from build123d import *

# Parameters (mm, degrees)
ESQUISSE1_W        = 265
ESQUISSE1_H        = 227
ESQUISSE1_R        = 6.5
ESQUISSE1_R_2      = 1.75
ESQUISSE1_R_3      = 1.749999999
ESQUISSE1_W_2      = 191
ESQUISSE1_H_2      = 156.859849262
ESQUISSE1_W_3      = 17
ESQUISSE1_H_3      = 80
BOSS_EXTRU_1_DEPTH = 6


with BuildPart() as part:
    # Esquisse1 → Boss.-Extru.1 (new body)
    with BuildSketch(Plane(origin=(0, 0, 0), x_dir=(1, 0, 0), z_dir=(0, 1, 0))):
        with Locations((132.5, -113.5)):
            Rectangle(ESQUISSE1_W, ESQUISSE1_H)
        with Locations(Location((246.5, -113.5, 0), (0, 0, 270))):
            Circle(ESQUISSE1_R, mode=Mode.SUBTRACT)
        with Locations(Location((246.5, -103.5, 0), (0, 0, 270))):
            Circle(ESQUISSE1_R_2, mode=Mode.SUBTRACT)
        with Locations(Location((253.571068024, -106.4289324, 0), (0, 0, 270))):
            Circle(ESQUISSE1_R_2, mode=Mode.SUBTRACT)
        with Locations(Location((256.5, -113.5, 0), (0, 0, 270))):
            Circle(ESQUISSE1_R_2, mode=Mode.SUBTRACT)
        with Locations(Location((253.571067812, -120.571067812, 0), (0, 0, 270))):
            Circle(ESQUISSE1_R_2, mode=Mode.SUBTRACT)
        with Locations(Location((246.5, -123.5, 0), (0, 0, 270))):
            Circle(ESQUISSE1_R_2, mode=Mode.SUBTRACT)
        with Locations(Location((239.428932188, -120.571067812, 0), (0, 0, 270))):
            Circle(ESQUISSE1_R_2, mode=Mode.SUBTRACT)
        with Locations(Location((236.5, -113.5, 0), (0, 0, 270))):
            Circle(ESQUISSE1_R_2, mode=Mode.SUBTRACT)
        with Locations(Location((239.42893238, -106.428931957, 0), (0, 0, 270))):
            Circle(ESQUISSE1_R_3, mode=Mode.SUBTRACT)
        with Locations(Location((259.935029054, -100.064971369, 0), (0, 0, 270))):
            Circle(ESQUISSE1_R_2, mode=Mode.SUBTRACT)
        with Locations(Location((259.935028843, -126.935028843, 0), (0, 0, 270))):
            Circle(ESQUISSE1_R_2, mode=Mode.SUBTRACT)
        with Locations(Location((233.064971369, -100.064970946, 0), (0, 0, 270))):
            Circle(ESQUISSE1_R_2, mode=Mode.SUBTRACT)
        with Locations(Location((233.064971157, -126.935028843, 0), (0, 0, 270))):
            Circle(ESQUISSE1_R_2, mode=Mode.SUBTRACT)
        with Locations(Location((132.5, -209.464962315, 0), (0, 0, 270))):
            Circle(ESQUISSE1_R, mode=Mode.SUBTRACT)
        with Locations(Location((132.5, -199.464962315, 0), (0, 0, 270))):
            Circle(ESQUISSE1_R_2, mode=Mode.SUBTRACT)
        with Locations(Location((139.571068024, -202.393894715, 0), (0, 0, 270))):
            Circle(ESQUISSE1_R_2, mode=Mode.SUBTRACT)
        with Locations(Location((142.5, -209.464962315, 0), (0, 0, 270))):
            Circle(ESQUISSE1_R_2, mode=Mode.SUBTRACT)
        with Locations(Location((139.571067812, -216.536030127, 0), (0, 0, 270))):
            Circle(ESQUISSE1_R_2, mode=Mode.SUBTRACT)
        with Locations(Location((132.5, -219.464962315, 0), (0, 0, 270))):
            Circle(ESQUISSE1_R_2, mode=Mode.SUBTRACT)
        with Locations(Location((125.428932188, -216.536030127, 0), (0, 0, 270))):
            Circle(ESQUISSE1_R_2, mode=Mode.SUBTRACT)
        with Locations(Location((122.5, -209.464962315, 0), (0, 0, 270))):
            Circle(ESQUISSE1_R_2, mode=Mode.SUBTRACT)
        with Locations(Location((125.42893238, -202.393894272, 0), (0, 0, 270))):
            Circle(ESQUISSE1_R_3, mode=Mode.SUBTRACT)
        with Locations(Location((145.935029054, -196.029933685, 0), (0, 0, 270))):
            Circle(ESQUISSE1_R_2, mode=Mode.SUBTRACT)
        with Locations(Location((145.935028843, -222.899991158, 0), (0, 0, 270))):
            Circle(ESQUISSE1_R_2, mode=Mode.SUBTRACT)
        with Locations(Location((119.064971369, -196.029933261, 0), (0, 0, 270))):
            Circle(ESQUISSE1_R_2, mode=Mode.SUBTRACT)
        with Locations(Location((119.064971157, -222.899991158, 0), (0, 0, 270))):
            Circle(ESQUISSE1_R_2, mode=Mode.SUBTRACT)
        with Locations(Location((18.513965978, -113.5, 0), (0, 0, 270))):
            Circle(ESQUISSE1_R, mode=Mode.SUBTRACT)
        with Locations(Location((18.513965978, -103.5, 0), (0, 0, 270))):
            Circle(ESQUISSE1_R_2, mode=Mode.SUBTRACT)
        with Locations(Location((25.585034002, -106.4289324, 0), (0, 0, 270))):
            Circle(ESQUISSE1_R_2, mode=Mode.SUBTRACT)
        with Locations(Location((28.513965978, -113.5, 0), (0, 0, 270))):
            Circle(ESQUISSE1_R_2, mode=Mode.SUBTRACT)
        with Locations(Location((25.58503379, -120.571067812, 0), (0, 0, 270))):
            Circle(ESQUISSE1_R_2, mode=Mode.SUBTRACT)
        with Locations(Location((18.513965978, -123.5, 0), (0, 0, 270))):
            Circle(ESQUISSE1_R_2, mode=Mode.SUBTRACT)
        with Locations(Location((11.442898166, -120.571067812, 0), (0, 0, 270))):
            Circle(ESQUISSE1_R_2, mode=Mode.SUBTRACT)
        with Locations(Location((8.513965978, -113.5, 0), (0, 0, 270))):
            Circle(ESQUISSE1_R_2, mode=Mode.SUBTRACT)
        with Locations(Location((11.442898358, -106.428931957, 0), (0, 0, 270))):
            Circle(ESQUISSE1_R_3, mode=Mode.SUBTRACT)
        with Locations(Location((31.948995033, -100.064971369, 0), (0, 0, 270))):
            Circle(ESQUISSE1_R_2, mode=Mode.SUBTRACT)
        with Locations(Location((31.948994821, -126.935028843, 0), (0, 0, 270))):
            Circle(ESQUISSE1_R_2, mode=Mode.SUBTRACT)
        with Locations(Location((5.078937347, -100.064970946, 0), (0, 0, 270))):
            Circle(ESQUISSE1_R_2, mode=Mode.SUBTRACT)
        with Locations(Location((5.078937136, -126.935028843, 0), (0, 0, 270))):
            Circle(ESQUISSE1_R_2, mode=Mode.SUBTRACT)
        with Locations(Location((132.5, -18.5, 0), (0, 0, 270))):
            Circle(ESQUISSE1_R, mode=Mode.SUBTRACT)
        with Locations(Location((132.5, -8.5, 0), (0, 0, 270))):
            Circle(ESQUISSE1_R_2, mode=Mode.SUBTRACT)
        with Locations(Location((139.571068024, -11.4289324, 0), (0, 0, 270))):
            Circle(ESQUISSE1_R_2, mode=Mode.SUBTRACT)
        with Locations(Location((142.5, -18.5, 0), (0, 0, 270))):
            Circle(ESQUISSE1_R_2, mode=Mode.SUBTRACT)
        with Locations(Location((139.571067812, -25.571067812, 0), (0, 0, 270))):
            Circle(ESQUISSE1_R_2, mode=Mode.SUBTRACT)
        with Locations(Location((132.5, -28.5, 0), (0, 0, 270))):
            Circle(ESQUISSE1_R_2, mode=Mode.SUBTRACT)
        with Locations(Location((125.428932188, -25.571067812, 0), (0, 0, 270))):
            Circle(ESQUISSE1_R_2, mode=Mode.SUBTRACT)
        with Locations(Location((122.5, -18.5, 0), (0, 0, 270))):
            Circle(ESQUISSE1_R_2, mode=Mode.SUBTRACT)
        with Locations(Location((125.42893238, -11.428931957, 0), (0, 0, 270))):
            Circle(ESQUISSE1_R_3, mode=Mode.SUBTRACT)
        with Locations(Location((145.935029054, -5.064971369, 0), (0, 0, 270))):
            Circle(ESQUISSE1_R_2, mode=Mode.SUBTRACT)
        with Locations(Location((145.935028843, -31.935028843, 0), (0, 0, 270))):
            Circle(ESQUISSE1_R_2, mode=Mode.SUBTRACT)
        with Locations(Location((119.064971369, -5.064970946, 0), (0, 0, 270))):
            Circle(ESQUISSE1_R_2, mode=Mode.SUBTRACT)
        with Locations(Location((119.064971157, -31.935028843, 0), (0, 0, 270))):
            Circle(ESQUISSE1_R_2, mode=Mode.SUBTRACT)
        with Locations(Location((260, -5, 0), (0, 0, 270))):
            Circle(ESQUISSE1_R_2, mode=Mode.SUBTRACT)
        with Locations(Location((233.064971369, -5, 0), (0, 0, 270))):
            Circle(ESQUISSE1_R_2, mode=Mode.SUBTRACT)
        with Locations(Location((260, -222, 0), (0, 0, 90))):
            Circle(ESQUISSE1_R_2, mode=Mode.SUBTRACT)
        with Locations(Location((233.064971369, -222, 0), (0, 0, 90))):
            Circle(ESQUISSE1_R_2, mode=Mode.SUBTRACT)
        with Locations(Location((5, -5, 0), (0, 0, 90))):
            Circle(ESQUISSE1_R_2, mode=Mode.SUBTRACT)
        with Locations(Location((31.935028631, -5, 0), (0, 0, 90))):
            Circle(ESQUISSE1_R_2, mode=Mode.SUBTRACT)
        with Locations(Location((5, -222, 0), (0, 0, 270))):
            Circle(ESQUISSE1_R_2, mode=Mode.SUBTRACT)
        with Locations(Location((31.935028631, -222, 0), (0, 0, 270))):
            Circle(ESQUISSE1_R_2, mode=Mode.SUBTRACT)
        with Locations((132.5, -113.5)):
            Rectangle(ESQUISSE1_W_2, ESQUISSE1_H_2, mode=Mode.SUBTRACT)
        with Locations((246.5, -58)):
            Rectangle(ESQUISSE1_W_3, ESQUISSE1_H_3, mode=Mode.SUBTRACT)
        with Locations((246.5, -169)):
            Rectangle(ESQUISSE1_W_3, ESQUISSE1_H_3, mode=Mode.SUBTRACT)
        with Locations((18.5, -58)):
            Rectangle(ESQUISSE1_W_3, ESQUISSE1_H_3, mode=Mode.SUBTRACT)
        with Locations((18.5, -169)):
            Rectangle(ESQUISSE1_W_3, ESQUISSE1_H_3, mode=Mode.SUBTRACT)
    extrude(amount=BOSS_EXTRU_1_DEPTH)


solid = part.part
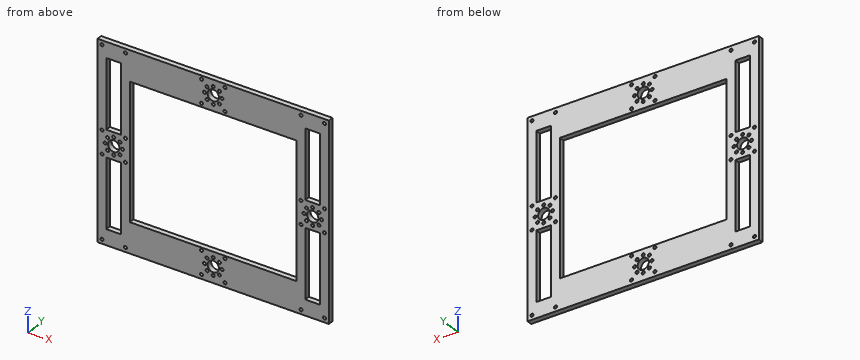
For this review, take the finished solid that the model builds, in its own axes (mm). Give positions to 0.01 mm unless a question says otherwise; leave off trailing zeros. Order: outer loops, then holes, each group sorted by start corner. A loop starts at its lowest first (then second) coordinate and runs counter-clockwise, first axis right, second up. Notation, with made-up numbers: (72, 27) - (79, 27) arc R20 cw to (79, 63) - close; hole circle Ø5 at (11, 41.5). An arc over 180 degrees is marked (long way). Answer as a JSON object with one key per item and string values. Group by question number.
Item 1: Wall thickness on line 1 along X through (y, z) = (1.7, 134); line 2 along X through (y, z) = (2.6, 123.5); line 3 along X through (y, z) = (2.7, 26): over which ranges is each line inside the solid? List them lowest first.
Item 2: Clearance check with a flat-ended pin moving along its axis: pin 1 Ø3 at (x, z) = (233.06, 5) entering from -Y. State where the tip first meets the part, or that it passes through.
Item 3: Take a section at B-B on x = 151. Give the boundary of the cut face in (y, z).
Item 4: Take a section at A-A on z = 64.5. Give the boundary of the cut face in (x, y).
Item 5: Take a section at C-C on y = 3.4. Give the number of separate pieces and of enclosed holes in the cut face, and give its area (3 significant figures).
Reported:
{
 "1": {"line 1": "0 to 10, 27 to 37, 228 to 238, 255 to 265", "line 2": "0 to 16.76, 20.26 to 37, 228 to 244.75, 248.25 to 265", "line 3": "0 to 10, 27 to 123.73, 127.13 to 137.87, 141.27 to 238, 255 to 265"},
 "2": {"pin 1": "through"},
 "3": {"outline": "(0, 0) - (6, 0) - (6, 35.07) - (0, 35.07) - close; (0, 191.93) - (6, 191.93) - (6, 227) - (0, 227) - close"},
 "4": {"outline": "(0, 0) - (10, 0) - (10, 6) - (0, 6) - close; (27, 0) - (37, 0) - (37, 6) - (27, 6) - close; (228, 0) - (238, 0) - (238, 6) - (228, 6) - close; (255, 0) - (265, 0) - (265, 6) - (255, 6) - close"},
 "5": {"separate pieces": "1", "enclosed holes": "65", "area": "23,700 mm^2"}
}
